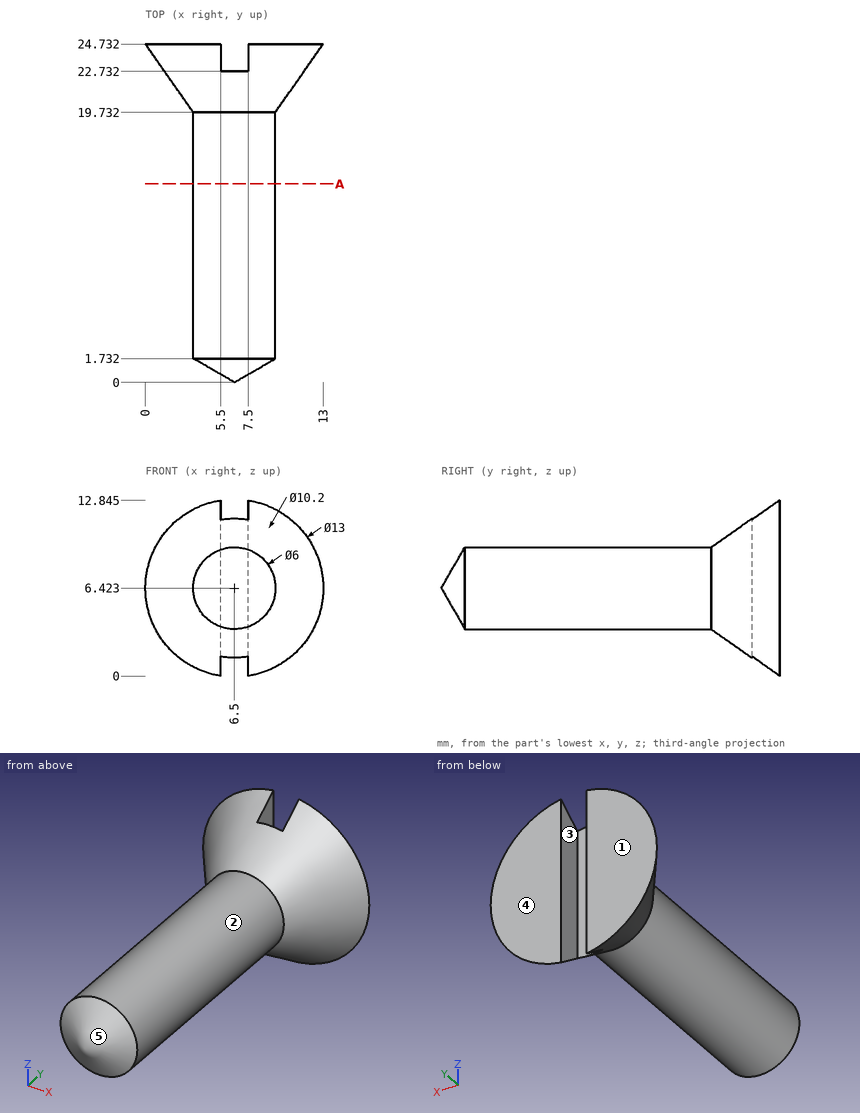
Drawing for the job (mm, zero at the part's lowest x, y, z). A direction names the side the tool comes from. Coordinates: 2 decimals unless noted, no trailing zeros. Loops run counter-clockwise (first coordinate to the right, second up) from the corner with the lowest first, then second, coordinate; pieces in that order, holes last. Notation, with made-up numbers: (75, -40) - (119, -40) arc R26 cw to (119, -14) - close; hole circle Ø9 at (62, 11). An arc over 180 degrees is marked (long way). Use CSV: the item, a comma, the result in double quotes. Start each with the question number.
Q1. Drop flat-ended pins along their axis: P1, Ø5, axis at y = 11.5, z = 9, coming from the +X side; P2, Ø5, axis at x = 4.5, y = 10, coming from the +Z side; P3, Ø1.6, axis at y = 23.5, z = 8.5, coming from the -X side (1 decimal); P4, Ø1, axis at y = 17, z = 11, coming from the -X side. Give the stop position or say it passes through.
Q2. 3-axis set-ups, long thin cutter, end or side, ignore diameter. For the marked faces 1 and 2: which of +Z, -Z, +X, -X, +Y, -Y reach the whole face in a straight line?
Q3. Two-plate mould, pull along X, no slides. Class the marked faces 3, 4 and 5: +X half, -X half, draft (parallel to the pull), parting line (faces both ways), or undercut.
Q4. Probe probe 1 along X at (y, z) = (12.25, 6.5); probe 2 along Z at (x, y) = (7.5, 22.5); probe 3 along Z at (x, y) = (6.5, 16.5). List the from-to ranges inside material, lowest first. Write a range as from..to.
Q5. Cut at A-A, the plane y = 14.5. List the corners of the cut face in (x, z).
Here are the results:
1,P1,"x = 9.5"
1,P2,"z = 9.42"
1,P3,"x = 0.6"
1,P4,"through"
2,face 1,"+Z, -Z, +X, -X, +Y"
2,face 2,"-Y"
3,face 3,"undercut"
3,face 4,"draft"
3,face 5,"parting line"
4,probe 1,"3.5..9.5"
4,probe 2,"1.59..11.26"
4,probe 3,"3.42..9.42"
5,outline,"circle Ø6 at (6.5, 6.42)"
